Here's how the part is built. I have some questions about the finished solid (model axes, mm). Round coordinates to 2 decimals unless told otherwise and drop trailing zeros. One line per question, with ' | ' between items. Start each with the question number.
(1) Will these pins go through, and if not, where does the flat tip stop? pin 1 (5 mm diameter, centred on x = -24, y = 83.25, fed in from +Z); pin 2 (1.5 mm diameter, centred on y = 58, z = 3, fed in from -X); pin 3 (5.5 mm diameter, centred on x = -24, y = 83.25, fed in from +Z).
(2) Imagine slicing it at A-A (z = 1.5). Give the number of separate pieces and of enclosed holes in the cut face, plus the area to 3 significant figures.
(3) If I drill on L1, parallel to Y at x = -72, z = 4.2; L2, parallel to Y at x = -40, z = 3.4; L3, parallel to X at y = 47, z = 3.8, over which ranges is the centre line in solid material (lowest first)?
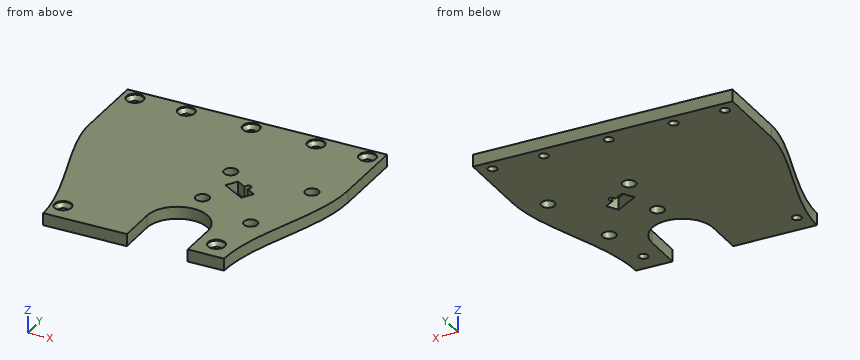
from build123d import *

# Parameters (mm, degrees)
SKETCH1_R                                    = 1.5
BOSS_EXTRUDE1_DEPTH                          = 4.5
SKETCH2_R                                    = 2.5
CUT_EXTRUDE1_DEPTH                           = 130.97115079
SKETCH3_R                                    = 1
CUT_EXTRUDE2_DEPTH                           = 130.97115079
CUT_EXTRUDE3_DEPTH                           = 130.97115079
CSK_FOR_M3_COUNTERSUNK_FLAT_HEAD_SCR_2_COUNT = 2
CSK_FOR_M3_COUNTERSUNK_FLAT_HEAD_SCR_2_PITCH = 19
CSK_FOR_M3_COUNTERSUNK_FLAT_HEAD_SCR_3_COUNT = 2
CSK_FOR_M3_COUNTERSUNK_FLAT_HEAD_SCR_3_PITCH = 43
CSK_FOR_M3_COUNTERSUNK_FLAT_HEAD_SCR_4_COUNT = 2
CSK_FOR_M3_COUNTERSUNK_FLAT_HEAD_SCR_4_PITCH = 67
CSK_FOR_M3_COUNTERSUNK_FLAT_HEAD_SCR_5_COUNT = 2
CSK_FOR_M3_COUNTERSUNK_FLAT_HEAD_SCR_5_PITCH = 86
CSK_FOR_M3_COUNTERSUNK_FLAT_HEAD_SCR_6_COUNT = 2
CSK_FOR_M3_COUNTERSUNK_FLAT_HEAD_SCR_6_PITCH = 102.971476633
CSK_FOR_M3_COUNTERSUNK_FLAT_HEAD_SCR_7_COUNT = 2
CSK_FOR_M3_COUNTERSUNK_FLAT_HEAD_SCR_7_PITCH = 76.857416688


with BuildPart() as part:
    # Sketch1 → Boss-Extrude1 (new body)
    with BuildSketch(Plane.XY):
        with BuildLine():
            Line((-96, 87.5), (0, 87.5))
            Line((0, 87.5), (0, 60))
            add(Edge.make_bspline(
                [(0, 60), (0, 47.440932757), (-8.740761153, 28.351955076), (-14.5, 8.088351659), (-14.5, 0)],
                knots=[0, 0, 0, 0, 0.602811114, 1, 1, 1, 1], degree=3))
            Line((-14.5, 0), (-28, 0))
            Line((-28, 0), (-28, 14.25))
            ThreePointArc((-28, 14.25), (-39.25, 25.5), (-50.5, 14.25))
            Line((-50.5, 14.25), (-50.5, 0))
            Line((-50.5, 0), (-81.5, 0))
            add(Edge.make_bspline(
                [(-96, 60), (-96, 44.479329369), (-81.5, 17.438131956), (-81.5, 0)],
                knots=[0, 0, 0, 0, 1, 1, 1, 1], degree=3))
            Line((-96, 60), (-96, 87.5))
        make_face()
        with Locations((-91, 83.25)):
            Circle(SKETCH1_R, mode=Mode.SUBTRACT)
        with Locations((-72, 83.25)):
            Circle(SKETCH1_R, mode=Mode.SUBTRACT)
        with Locations((-48, 83.25)):
            Circle(SKETCH1_R, mode=Mode.SUBTRACT)
        with Locations((-5, 83.25)):
            Circle(SKETCH1_R, mode=Mode.SUBTRACT)
        with Locations((-24, 83.25)):
            Circle(SKETCH1_R, mode=Mode.SUBTRACT)
        with Locations((-21.25, 7.5)):
            Circle(SKETCH1_R, mode=Mode.SUBTRACT)
        with Locations((-78, 7.5)):
            Circle(SKETCH1_R, mode=Mode.SUBTRACT)
    extrude(amount=BOSS_EXTRUDE1_DEPTH)

    # Sketch2 → Cut-Extrude1 (cut, through all)
    with BuildSketch(Plane.XY.offset(4.5)):
        with Locations((-10, 53.5)):
            Circle(SKETCH2_R)
        with Locations((-40, 53.5)):
            Circle(SKETCH2_R)
        with Locations((-40, 33.5)):
            Circle(SKETCH2_R)
        with Locations((-18, 25.5)):
            Circle(SKETCH2_R)
    extrude(amount=-CUT_EXTRUDE1_DEPTH, mode=Mode.SUBTRACT)

    # Sketch3 → Cut-Extrude2 (cut, through all)
    with BuildSketch(Plane.XY.offset(4.5)):
        with Locations((-30.001125718, 46.899563619)):
            Circle(SKETCH3_R)
    extrude(amount=-CUT_EXTRUDE2_DEPTH, mode=Mode.SUBTRACT)

    # Sketch4 → Cut-Extrude3 (cut, through all)
    with BuildSketch(Plane(origin=(0, 0, 0), x_dir=(-1, 0, 0), z_dir=(0, 0, -1))):
        with BuildLine():
            Line((28.728353494, 39.348401399), (37.282344284, 44.528096521))
            Line((37.282344284, 44.528096521), (34.796090626, 48.634012101))
            Line((34.796090626, 48.634012101), (31.37449431, 46.562134052))
            Line((31.37449431, 46.562134052), (30.856524797, 47.417533131))
            ThreePointArc((30.856524797, 47.417533131), (29.500195325, 47.765051192), (29.125889015, 46.415868763))
            Line((29.125889015, 46.415868763), (29.664366906, 45.526601189))
            Line((29.664366906, 45.526601189), (26.242099835, 43.454316978))
            Line((26.242099835, 43.454316978), (28.728353494, 39.348401399))
        make_face()
    extrude(amount=-CUT_EXTRUDE3_DEPTH, mode=Mode.SUBTRACT)

    # Sketch6 → CSK for M3 Countersunk Flat Head Screw1 (revolve, cut)
    with BuildSketch(Plane(origin=(-91, 83.25, 4.5), x_dir=(0, -1, 0), z_dir=(1, 0, 0))):
        Polygon((0, 0), (0, 4.5), (1.7, 4.5), (1.7, 1.85), (3.15, 0.4), (3.15, 0), align=None)
    csk_for_m3_countersunk_flat_head_screw1 = revolve(axis=Axis((-91, 83.25, 10.85), (0, 0, -1)), mode=Mode.SUBTRACT)

    # CSK for M3 Countersunk Flat Head Scr 2: CSK for M3 Countersunk Flat Head Screw1 ×2
    with Locations(*[(i * CSK_FOR_M3_COUNTERSUNK_FLAT_HEAD_SCR_2_PITCH, 0, 0) for i in range(1, CSK_FOR_M3_COUNTERSUNK_FLAT_HEAD_SCR_2_COUNT)]):
        add(csk_for_m3_countersunk_flat_head_screw1, mode=Mode.SUBTRACT)

    # CSK for M3 Countersunk Flat Head Scr 3: CSK for M3 Countersunk Flat Head Screw1 ×2
    with Locations(*[(i * CSK_FOR_M3_COUNTERSUNK_FLAT_HEAD_SCR_3_PITCH, 0, 0) for i in range(1, CSK_FOR_M3_COUNTERSUNK_FLAT_HEAD_SCR_3_COUNT)]):
        add(csk_for_m3_countersunk_flat_head_screw1, mode=Mode.SUBTRACT)

    # CSK for M3 Countersunk Flat Head Scr 4: CSK for M3 Countersunk Flat Head Screw1 ×2
    with Locations(*[(i * CSK_FOR_M3_COUNTERSUNK_FLAT_HEAD_SCR_4_PITCH, 0, 0) for i in range(1, CSK_FOR_M3_COUNTERSUNK_FLAT_HEAD_SCR_4_COUNT)]):
        add(csk_for_m3_countersunk_flat_head_screw1, mode=Mode.SUBTRACT)

    # CSK for M3 Countersunk Flat Head Scr 5: CSK for M3 Countersunk Flat Head Screw1 ×2
    with Locations(*[(i * CSK_FOR_M3_COUNTERSUNK_FLAT_HEAD_SCR_5_PITCH, 0, 0) for i in range(1, CSK_FOR_M3_COUNTERSUNK_FLAT_HEAD_SCR_5_COUNT)]):
        add(csk_for_m3_countersunk_flat_head_screw1, mode=Mode.SUBTRACT)

    # CSK for M3 Countersunk Flat Head Scr 6: CSK for M3 Countersunk Flat Head Screw1 ×2
    with Locations(*[Vector(0.6773720478781835, -0.7356406111365222, 0) * (i * CSK_FOR_M3_COUNTERSUNK_FLAT_HEAD_SCR_6_PITCH) for i in range(1, CSK_FOR_M3_COUNTERSUNK_FLAT_HEAD_SCR_6_COUNT)]):
        add(csk_for_m3_countersunk_flat_head_screw1, mode=Mode.SUBTRACT)

    # CSK for M3 Countersunk Flat Head Scr 7: CSK for M3 Countersunk Flat Head Screw1 ×2
    with Locations(*[Vector(0.1691443787750649, -0.9855912840162485, 0) * (i * CSK_FOR_M3_COUNTERSUNK_FLAT_HEAD_SCR_7_PITCH) for i in range(1, CSK_FOR_M3_COUNTERSUNK_FLAT_HEAD_SCR_7_COUNT)]):
        add(csk_for_m3_countersunk_flat_head_screw1, mode=Mode.SUBTRACT)


solid = part.part
Check sheet entries:
1) pin 1: z = 3.45 | pin 2: x = -95.97 | pin 3: z = 3.7
2) separate pieces: 1 | enclosed holes: 12 | area: 6,810 mm^2
3) L1: 0 to 80.1, 86.4 to 87.5 | L2: 25.47 to 31, 36 to 51, 56 to 87.5 | L3: -93.86 to -35.79, -32.1 to -31.11, -29.01 to -1.7
